from build123d import *

# Parameters (mm, degrees)
F0_R     = 304.8
F0_R_2   = 196.85
F1_DEPTH = 38.1
F2_R     = 304.8
F2_R_2   = 215.9889
F3_DEPTH = 63.5


with BuildPart() as f1:
    # F0 (on Front) → F1 (new body)
    with BuildSketch(Plane.XZ):
        Circle(F0_R)
        Circle(F0_R_2, mode=Mode.SUBTRACT)
    extrude(amount=F1_DEPTH)

    # F2 (on face) → F3 (join)
    with BuildSketch(Plane.XZ.offset(38.1)):
        Circle(F2_R)
        Circle(F2_R_2, mode=Mode.SUBTRACT)
    extrude(amount=F3_DEPTH)

    # F4: F1 across face


with BuildPart() as f1_1:
    add(f1.part)
    add(f1.part.mirror(Plane(origin=(0, 0, 0), x_dir=(1, 0, 0), z_dir=(0, 1, 0))))


solid = f1_1.part
Input: part model. Units: mm. Frame: model coordinates. A direction names the side the tool comes from. Give positions to 0.01 mm unless a question says otherwise; leave off trailing zeros. Order: outer loops, then holes, each group sorted by start corner. A loop starts at its lowest first (then second) coordinate and runs counter-clockwise, first axis right, second up. Notation, with made-up numbers: M -35,29.5 L -23,29.5 A16 ccw -23,39.5 Z; hole C -25.75,42.5 d4. An arc over 180 degrees is marked long. Answer as a JSON object with one key per item and string values.
1. Cut plane C-C, the plane y = 10.5. Output: boundary loops of the cut face in (x, z).
Result sheet:
{"outline": "C 0,0 d609.6; hole C 0,0 d393.7"}
2. Cut plane D-D, the plane z = -244.5. Output: boundary loops of the cut face in (x, y), and give its area (3 significant figures).
Result sheet:
{"outline": "M -182,-101.6 L 182,-101.6 L 182,101.6 L -182,101.6 Z", "area": "74,000 mm²"}
3. First-contact query: P1, Ø1.5, axis at x = 219.5, y = 72.5, coming from the +Z side; P2, Ø4, axis at x = -207, y = 5, coming from the -Z side; P3, Ø6, axis at y = 20.5, z = 135, coming from the +X side. Flat tips, straight axial feed; report the tip coordinate or a pass-through.
Result sheet:
{"P1": "z = 212.25", "P2": "z = -225.56", "P3": "x = 274.73"}
4. Cut plane A-A, the plane x = 0. Output: boundary loops of the cut face in (y, z), and give its area (3 significant figures).
Result sheet:
{"outline": "M -101.6,-304.8 L 101.6,-304.8 L 101.6,-215.99 L 38.1,-215.99 L 38.1,-196.85 L -38.1,-196.85 L -38.1,-215.99 L -101.6,-215.99 Z; M -101.6,215.99 L -38.1,215.99 L -38.1,196.85 L 38.1,196.85 L 38.1,215.99 L 101.6,215.99 L 101.6,304.8 L -101.6,304.8 Z", "area": "39,000 mm²"}
5. Cut plane B-B, the plane z = 0. Output: boundary loops of the cut face in (x, y), and give its area (3 significant figures).
Result sheet:
{"outline": "M -304.8,-101.6 L -215.99,-101.6 L -215.99,-38.1 L -196.85,-38.1 L -196.85,38.1 L -215.99,38.1 L -215.99,101.6 L -304.8,101.6 Z; M 196.85,-38.1 L 215.99,-38.1 L 215.99,-101.6 L 304.8,-101.6 L 304.8,101.6 L 215.99,101.6 L 215.99,38.1 L 196.85,38.1 Z", "area": "39,000 mm²"}
6. Reachability of faces 1 (the cylindrical face through (-241.879, -1.422, -185.466)), 2 (the cylindrical face through (-28.12, 69.41, 214.15)), 3 (the cylindrical face through (-28.12, -69.41, 214.15)) from +Z, -Z, +X, -X, +Y, -Y: full face, straight path, thin tool, end or side. Return the list, or none.
Result sheet:
{"face 1": "+Y, -Y", "face 2": "+Y", "face 3": "-Y"}
7. Ray query, line 1 (Z direction, x = 0, y = -73); line 2 (X direction, y = -52.5, z = 109); line 3 (X direction, y = -67, z = -188.5). Return the intervals inside material, ascending. Write a range as [from, to].
Result sheet:
{"line 1": "[-304.8, -215.99], [215.99, 304.8]", "line 2": "[-284.64, -186.47], [186.47, 284.64]", "line 3": "[-239.52, -105.45], [105.45, 239.52]"}
